Verification items for the finished model (mm, model axes). A direction names the side the tool comes from. Coordinates: 2 decimals unless noted, no trailing zeros. Order: outer loops, then holes, each group sorted by start corner. A loop starts at its lowest first (then second) coordinate and runs counter-clockwise, first axis right, second up. Notation, with made-up numbers: M 28,44.25 L 38,44.25 A18 ccw 38,74.25 Z; hole C 20.5,15 d11. An arc over 180 degrees is marked long. Use one line per item in the form item = value. Start each with the question number.
```python
from build123d import *

# Parameters (mm, degrees)
SKETCH1_R           = 33.905425059
BOSS_EXTRUDE1_DEPTH = 88
SKETCH2_R           = 10
CUT_REVOLVE1_ANGLE  = 180
FILLET1_R           = 5
CHAMFER1_SIZE       = 5


with BuildPart() as part:
    # Sketch1 → Boss-Extrude1 (new body)
    with BuildSketch(Plane(origin=(0, 0, 0), x_dir=(1, 0, 0), z_dir=(0, 1, 0))):
        with Locations(Location((0, 0, 0), (0, 0, 270))):
            Circle(SKETCH1_R)
    extrude(amount=BOSS_EXTRUDE1_DEPTH)

    # Sketch2 → Cut-Revolve1 (revolve, cut)
    with BuildSketch(Plane.XY):
        with Locations((33.905425059, 68)):
            Circle(SKETCH2_R)
        with Locations((-33.905425059, 20)):
            Circle(SKETCH2_R)
    revolve(axis=Axis((0, 39.08266512, 0), (0, -1, 0)), revolution_arc=CUT_REVOLVE1_ANGLE, mode=Mode.SUBTRACT)

    # Fillet1
    fillet1_edges = [part.edges().sort_by_distance(p)[0] for p in [
        (0, 88, -33.905425059),
    ]]
    fillet(fillet1_edges, radius=FILLET1_R)

    # Chamfer1
    chamfer1_edges = [part.edges().sort_by_distance(p)[0] for p in [
        (0, 0, -33.905425059),
    ]]
    chamfer(chamfer1_edges, length=CHAMFER1_SIZE)


solid = part.part
```
1. Depth check by flat-ended pin: P1, Ø2, axis at x = -8, y = 35.5, coming from the +Z side; P2, Ø8, axis at x = -31.5, y = 21.5, coming from the -Z side; P3, Ø10, axis at x = -5.5, y = 71, coming from the +Z side. Enter the tip coordinate at first touch or a pass-through.
2. Cross-section at A-A on x = 0. Enter the section's corners in (y, z).
3. Material ranges on line 1 along Y through (x, z) = (20, 21); line 2 along Y through (x, z) = (-7, -25.5); line 3 along X through (y, z) = (24.5, -14), recorded low to high.
4. Cross-section at C-C on y = 69. Enter the section's corners in (x, z).
5. Release check for a two-part mould opening along Y. For faces 5 (the flat face through (0, 0, 0)), 6 (the flat face through (0, 88, 0)), 7 (the flat face through (-30, 68, 0)) record: pulls with the +Y half, pulls with the -Y half, needs draft (parallel to the pull), parting line crosses it, or undercut.
6. Cross-section at B-B on y = 33.5. Enter the section's corners in (x, z), and give its area (3 significant figures).
7. Tool access check on faces 1 (the flat face through (30, 68, 0)), 2 (the flat face through (30, 20, 0)), 3 (the conical face through (-11.164, 0.243, 26.926)), 4 (the flat face through (-30, 20, 0)). Record the directions out of +Z, -Z, +X, -X, +Y, -Y that give a thin tool (end or side, any length) a straight path to the whole face; none if there is none.
Final values:
q1.P1 = 33.17
q1.P2 = 0
q1.P3 = 27.42
q2.outline = M 0,-28.91 L 5,-33.91 L 10,-33.91 A10 cw 30,-33.91 L 83,-33.91 A5 ccw 88,-28.91 L 88,28.91 A5 ccw 83,33.91 L 78,33.91 A10 cw 58,33.91 L 5,33.91 L 0,28.91 Z
q3.line_1 = 0.09 to 59.29, 76.71 to 88
q3.line_2 = 0 to 13.34, 26.66 to 88
q3.line_3 = -20.68 to 20.68
q4.outline = M -33.91,0 A33.91 ccw 33.91,0 L 23.96,0 A23.96 ccw -23.96,0 Z
q5.face_5 = pulls with the -Y half
q5.face_6 = pulls with the +Y half
q5.face_7 = undercut
q6.outline = C 0,0 d67.81
q6.area = 3,610 mm2
q7.face_1 = +Z, +X
q7.face_2 = -Z, +X
q7.face_3 = -Y
q7.face_4 = -Z, -X
